```python
from build123d import *

# Parameters (mm, degrees)
F0_W     = 59.69
F0_H     = 59.69
F1_DEPTH = 37.58946
F2_R     = 15.24
F3_DEPTH = 37.59046
F5_DEPTH = 59.691
F7_D     = 5.5


with BuildPart() as f1:
    # F0 (on Front) → F1 (new body)
    with BuildSketch(Plane.XZ):
        Rectangle(F0_W, F0_H)
    extrude(amount=F1_DEPTH)

    # F2 (on face) → F3 (cut, through all)
    with BuildSketch(Plane.XZ.offset(37.58946)):
        Circle(F2_R)
    extrude(amount=-F3_DEPTH, mode=Mode.SUBTRACT)

    # F4 (on face) → F5 (cut, through all)
    with BuildSketch(Plane.XY.offset(29.845)):
        Polygon((-29.845, -12.7), (-17.145, 0), (-29.845, 0), align=None)
        Polygon((29.845, -12.7), (29.845, 0), (17.145, 0), align=None)
    extrude(amount=-F5_DEPTH, mode=Mode.SUBTRACT)

    # F7 (through all)
    with Locations(Plane.XZ.offset(37.58946)):
        with Locations((-23.49246, 23.49246), (23.49246, 23.49246), (23.49246, -23.49246), (-23.49246, -23.49246)):
            Hole(F7_D / 2)


solid = f1.part
```
Geometry: final body of the model. Coordinates: model frame, mm. Round coordinates to 2 decimals unless told otherwise and drop trailing zeros. Order: outer loops, then holes, each group sorted by start corner. A loop starts at its lowest first (then second) coordinate and runs counter-clockwise, first axis right, second up. Notation, with made-up numbers: M 23.5,-4.75 L 81.5,-4.75 A25 cw 81.5,21.25 Z; hole C 67.5,52.25 d9. An arc over 180 degrees is marked long. One line per item, written item: value.
(1) Pin query (flat end, axial travel): P1, Ø10, axis at y = -6, z = -10.5, coming from the +X side (3 decimals). Return the tip coordinate at first contact, or that it passes through.
Result sheet:
P1: x = 28.145
(2) Line query: probe 1 along X at (y, z) = (-10, 23) (3 decimals); probe 2 along Z at (x, y) = (22.5, -8) (3 decimals); probe 3 along Z at (x, y) = (0, -12.5) (3 decimals). Output: solid intervals per line, ascending. Write a range as [from, to].
Result sheet:
probe 1: [-27.145, -26.198], [-20.787, 20.787], [26.198, 27.145]
probe 2: [-29.845, -26.057], [-20.928, 20.928], [26.057, 29.845]
probe 3: [-29.845, -15.24], [15.24, 29.845]
(3) Pull-direction query (X, two-part tool) for faces 1 (the flat face through (0, -19, -29.845)), 2 (the flat face through (-29.845, -25, 0)), 3 (the cylindrical face through (20.95, -20.36, 22.44)); classes: pulls with the +X half, pulls with the -X half, needs draft (parallel to the pull), parting line crosses it, or undercut.
Result sheet:
face 1: needs draft
face 2: pulls with the -X half
face 3: undercut
(4) Cut plane C-C (y = -27). Return the cut outline in (x, z) (3 decimals).
Result sheet:
outline: M -29.845,-29.845 L 29.845,-29.845 L 29.845,29.845 L -29.845,29.845 Z; hole C -23.492,-23.492 d5.5; hole C -23.492,23.492 d5.5; hole C 0,0 d30.48; hole C 23.492,-23.492 d5.5; hole C 23.492,23.492 d5.5
(5) Cut plane B-B (z = 5). Return the cut outline in (x, y) (3 decimals).
Result sheet:
outline: M -29.845,-37.589 L -14.396,-37.589 L -14.396,0 L -17.145,0 L -29.845,-12.7 Z; M 14.396,-37.589 L 29.845,-37.589 L 29.845,-12.7 L 17.145,0 L 14.396,0 Z
(6) Cut plane A-A (x = 0). Return the cut outline in (y, z) (3 decimals), and give its area (3 significant figures).
Result sheet:
outline: M -37.589,-29.845 L 0,-29.845 L 0,-15.24 L -37.589,-15.24 Z; M -37.589,15.24 L 0,15.24 L 0,29.845 L -37.589,29.845 Z
area: 1,100 mm2
(7) Cut plane D-D (z = 16.5). Return the cut outline in (x, y) (3 decimals).
Result sheet:
outline: M -29.845,-37.589 L 29.845,-37.589 L 29.845,-12.7 L 17.145,0 L -17.145,0 L -29.845,-12.7 Z
